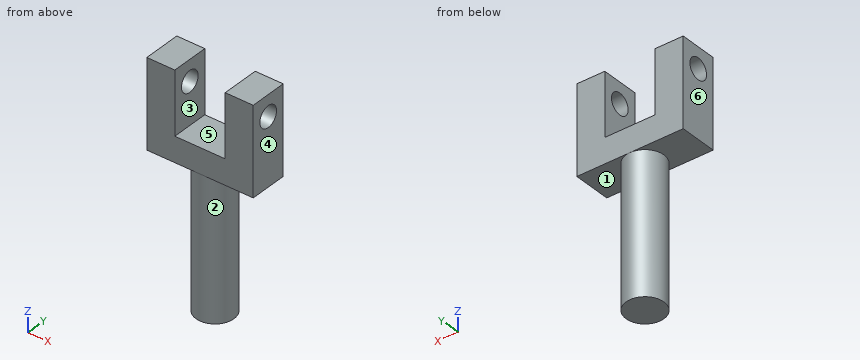
```python
from build123d import *

# Parameters (mm, degrees)
SKETCH1_R                = 1.35
BOSS_EXTRUDE1_DEPTH      = 10
BOSS_EXTRUDE5_DEPTH      = 1.35
BOSS_EXTRUDE5_DEPTH_BACK = 1.35
CUT_EXTRUDE1_DEPTH       = 11.25
CUT_EXTRUDE1_DEPTH_BACK  = 11.25
SKETCH4_R                = 0.75


with BuildPart() as part:
    # Sketch1 → Boss-Extrude1 (new body)
    with BuildSketch(Plane.XY):
        Circle(SKETCH1_R)
    extrude(amount=BOSS_EXTRUDE1_DEPTH)

    # Sketch3 → Boss-Extrude5 (add, two sides: drawn at the far end of the back side and taken through both)
    with BuildSketch(Plane(origin=(0, 0, 0), x_dir=(1, 0, 0), z_dir=(0, 1, 0)).offset(-BOSS_EXTRUDE5_DEPTH_BACK)):
        Polygon((0, -10), (-3.8, -10), (-3.8, -16.3), (-1.8, -16.3), (-1.8, -11.8), (1.8, -11.8), (1.8, -16.3), (3.8, -16.3), (3.8, -10), align=None)
    extrude(amount=BOSS_EXTRUDE5_DEPTH + BOSS_EXTRUDE5_DEPTH_BACK)

    # Sketch4 → Cut-Extrude1 (cut, two sides: drawn at the far end of the back side and taken through both)
    with BuildSketch(Plane(origin=(-1.8, 0, 0), x_dir=(0, 0, -1), z_dir=(1, 0, 0)).offset(-CUT_EXTRUDE1_DEPTH_BACK)):
        with Locations(Location((-14.8, 0, 0), (0, 0, 180))):
            Circle(SKETCH4_R)
    extrude(amount=CUT_EXTRUDE1_DEPTH + CUT_EXTRUDE1_DEPTH_BACK, mode=Mode.SUBTRACT)


solid = part.part
```
Geometry: final body of the model. Coordinates: model frame, mm. Face numbers are marked on the shaded views. A direction names the side the tool comes from. Give positions to 0.01 mm unless a question says otherwise; leave off trailing zeros. Loops run counter-clockwise (first coordinate to the right, second up) from the corner with the lowest first, then second, coordinate; pieces in that order, holes last. Notation, with made-up numbers: (19.25, -14.5) -> (54.25, -14.5) arc R22 cw to (54.25, 4.5) -> close; hole circle Ø4 at (-35, -36). An arc over 180 degrees is marked (long way). Return JSON: item names as keys, results as strings.
Item 1: Access query for the marked faces 5 and 6. Directions: +Z, -Z, +X, -X, +Y, -Y. A direction counts if a zero-diameter tool reaches every point of the face in a straight line with its end or side. Return the directions, or none.
Filled in:
{"face 5": "+Z, +Y, -Y", "face 6": "+Z, -Z, -X, +Y, -Y"}
Item 2: Section A-A, the plane y = 0. Output: boundary loops of the cut face in (x, z), plus the area to 3 significant figures.
Filled in:
{"outline": "(-3.8, 10) -> (-1.35, 10) -> (-1.35, 0) -> (1.35, 0) -> (1.35, 10) -> (3.8, 10) -> (3.8, 14.05) -> (1.8, 14.05) -> (1.8, 11.8) -> (-1.8, 11.8) -> (-1.8, 14.05) -> (-3.8, 14.05) -> close; (-3.8, 15.55) -> (-1.8, 15.55) -> (-1.8, 16.3) -> (-3.8, 16.3) -> close; (1.8, 15.55) -> (3.8, 15.55) -> (3.8, 16.3) -> (1.8, 16.3) -> close", "area": "52.7 mm^2"}
Item 3: Section B-B, the plane x = -2. Output: boundary loops of the cut face in (y, z).
Filled in:
{"outline": "(-1.35, 10) -> (1.35, 10) -> (1.35, 16.3) -> (-1.35, 16.3) -> close; hole circle Ø1.5 at (0, 14.8)"}
Item 4: Line query: line 1 (X direction, y = -0.8, z = 13.25); line 2 (Y direction, x = 3.05, z = 14.8); line 3 (Z direction, x = -1.5, y = -0.85). Output: solid intervals per line, ascending.
Filled in:
{"line 1": "-3.8 to -1.8, 1.8 to 3.8", "line 2": "-1.35 to -0.75, 0.75 to 1.35", "line 3": "10 to 11.8"}
Item 5: Section D-D, the plane x = 0.5. Output: boundary loops of the cut face in (y, z).
Filled in:
{"outline": "(-1.35, 10) -> (-1.25, 10) -> (-1.25, 0) -> (1.25, 0) -> (1.25, 10) -> (1.35, 10) -> (1.35, 11.8) -> (-1.35, 11.8) -> close"}
Item 6: Section C-C, the plane y = -1. Output: boundary loops of the cut face in (x, z), plus the area to 3 significant figures.
Filled in:
{"outline": "(-3.8, 10) -> (-0.91, 10) -> (-0.91, 0) -> (0.91, 0) -> (0.91, 10) -> (3.8, 10) -> (3.8, 16.3) -> (1.8, 16.3) -> (1.8, 11.8) -> (-1.8, 11.8) -> (-1.8, 16.3) -> (-3.8, 16.3) -> close", "area": "49.8 mm^2"}
Item 7: Pin query (flat end, axial travel): P1, Ø1.5, axis at y = 0.5, z = 3.5, coming from the +X side; P2, Ø1.4, axis at x = -0.5, y = 0.5, coming from the +Z side; P3, Ø0.8, axis at x = -2, y = -0.5, coming from the -Z side; P4, Ø1, axis at x = 2, z = 3.5, coming from the +Y side. Return the tip coordinate at first contact, or that it passes through.
Filled in:
{"P1": "x = 1.35", "P2": "z = 11.8", "P3": "z = 10", "P4": "through"}
Item 8: Mould query, pull axis X, two halves, no side actions, for the marked faces 1, 2, 3 and 4. Classes: released by +X, released by -X, zero draft, split by the parting line, or undercut.
Filled in:
{"face 1": "zero draft", "face 2": "split by the parting line", "face 3": "undercut", "face 4": "released by +X"}
